Could you check a few things on this model? Use its own coordinates, in mm. Face numbers are marked on the shaded views. Round coordinates to 2 decimals unless told otherwise and drop trailing zeros. Loops run counter-clockwise (first coordinate to the right, second up) from the corner with the lowest first, then second, coordinate; pieces in that order, holes last.
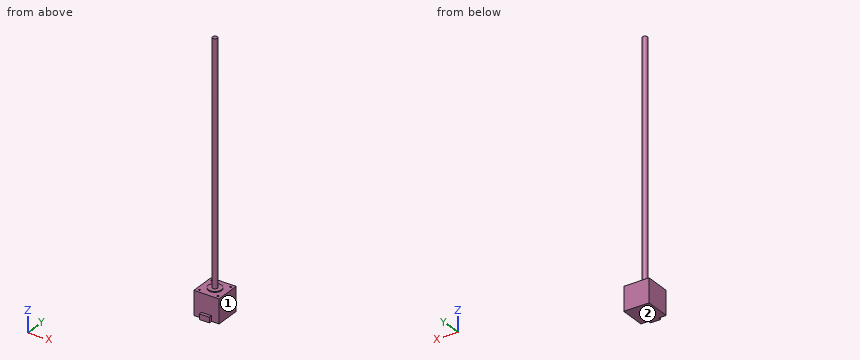
from build123d import *

# Parameters (mm, degrees)
SKETCH1_W           = 42.3
SKETCH1_H           = 42.3
BOSS_EXTRUDE1_DEPTH = 40
SKETCH1_3_R         = 1.5
CUT_EXTRUDE1_DEPTH  = 5
SKETCH1_4_R         = 11.25
SKETCH1_4_R_2       = 4
BOSS_EXTRUDE2_DEPTH = 1.5
SKETCH1_5_R         = 4
BOSS_EXTRUDE3_DEPTH = 400
SKETCH3_W           = 17
SKETCH3_H           = 9
BOSS_EXTRUDE4_DEPTH = 5


with BuildPart() as part:
    # Sketch1 → Boss-Extrude1 (new body)
    with BuildSketch(Plane.XY):
        Rectangle(SKETCH1_W, SKETCH1_H)
    extrude(amount=-BOSS_EXTRUDE1_DEPTH)

    # Sketch1<3> → Cut-Extrude1 (cut)
    with BuildSketch(Plane.XY):
        with Locations((-15.5, -15.5)):
            Circle(SKETCH1_3_R)
        with Locations((15.5, 15.5)):
            Circle(SKETCH1_3_R)
        with Locations((15.5, -15.5)):
            Circle(SKETCH1_3_R)
        with Locations((-15.5, 15.5)):
            Circle(SKETCH1_3_R)
    extrude(amount=-CUT_EXTRUDE1_DEPTH, mode=Mode.SUBTRACT)

    # Sketch1<4> → Boss-Extrude2 (add)
    with BuildSketch(Plane.XY):
        Circle(SKETCH1_4_R)
        Circle(SKETCH1_4_R_2, mode=Mode.SUBTRACT)
    extrude(amount=BOSS_EXTRUDE2_DEPTH)

    # Sketch1<5> → Boss-Extrude3 (add)
    with BuildSketch(Plane.XY):
        Circle(SKETCH1_5_R)
    extrude(amount=BOSS_EXTRUDE3_DEPTH)

    # Sketch3 → Boss-Extrude4 (add)
    with BuildSketch(Plane.XZ.offset(21.15)):
        with Locations((0, -35.5)):
            Rectangle(SKETCH3_W, SKETCH3_H)
    extrude(amount=BOSS_EXTRUDE4_DEPTH)


solid = part.part
Item 1: Will these pins go through, and if not, where does the flat tip stop? pin 1 (3.5 mm diameter, centred on x = -15.5, y = -16, fed in from +Z); pin 2 (1.5 mm diameter, centred on x = -4, y = -23, fed in from +Z); pin 3 (3 mm diameter, centred on x = 4.5, z = 278, fed in from -Y); pin 4 (10 mm diameter, centred on x = 12.5, z = 29, fed in from +Y).
Results list:
pin 1: stops at z = 0
pin 2: stops at z = -31
pin 3: stops at y = -2.65
pin 4: passes through
Item 2: If we section it at C-C, the plane z = 10: Please give me the cut outline in (x, y), then the cut area to 3 significant figures.
Results list:
outline: circle Ø8 at (0, 0)
area: 50.3 mm2
Item 3: If we section it at B-B, the plane x = 0: Please give me the cut outline in (y, z), then the cut area to 3 significant figures.
Results list:
outline: (-26.15, -40) - (21.15, -40) - (21.15, 0) - (11.25, 0) - (11.25, 1.5) - (4, 1.5) - (4, 400) - (-4, 400) - (-4, 1.5) - (-11.25, 1.5) - (-11.25, 0) - (-21.15, 0) - (-21.15, -31) - (-26.15, -31) - close
area: 4,960 mm2
Item 4: If we section it at A-A, the plane y = 0: Please give me the cut outline in (x, z).
Results list:
outline: (-21.15, -40) - (21.15, -40) - (21.15, 0) - (11.25, 0) - (11.25, 1.5) - (4, 1.5) - (4, 400) - (-4, 400) - (-4, 1.5) - (-11.25, 1.5) - (-11.25, 0) - (-21.15, 0) - close
Item 5: We'd pull the mould along Z, two halves only. Please class the marked faces 1 and 2: released by +Z, released by -Z, zero draft, split by the parting line, or undercut.
Results list:
face 1: zero draft
face 2: released by -Z
Item 6: If I drill on line 1 along Y through (x, z) = (15.5, -3.65); line 2 along Y through (x, z) = (-15, -1), over which ranges is the centre line in solid material (lowest first)?
Results list:
line 1: y = -21.15 to -17, -14 to 14, 17 to 21.15
line 2: y = -21.15 to -16.91, -14.09 to 14.09, 16.91 to 21.15
